Here's how the part is built. I have some questions about the finished solid (model axes, mm). Face numbers are marked on the shaded views. A direction names the side the tool comes from. Round coordinates to 2 decimals unless told otherwise and drop trailing zeros. Write each loop counter-clockwise with the first axis right and the second up, starting at its lowest first coordinate (ties: lowest second). Pieces come first, ordered by that corner, then holes. Notation, with made-up numbers: (38, 25) - (94, 25) arc R31 ccw to (94, 54) - close; hole circle Ø5 at (-11, -24.75). An arc over 180 degrees is marked (long way). Use one line per item in the form item = value. Start each with the question number.
1. Will this pin go through, and if not, where does the flat tip stop? pin 1 (10 mm diameter, centred on x = 6.5, z = 16, fed in from +Y).
2. Which directions (+Z, -Z, +X, -X, +Y, -Y) give clear straight access to the entire face, cutting with the end or side of a thin tool? Please do the marked faces 4 and 5.
3. I want a section at B-B, the plane z = 6. List the corners of the cut face in (x, y) for me.
4. I want a section at C-C, the plane x = -8.5. List the corners of the cut face in (y, z) for me, plus the area to 3 significant figures.
5. If I drill on line 1 along Z through (x, y) = (-1, 27), over which ranges is the centre line in solid material (lowest first)?
6. I want a section at D-D, the plane y = -30.5. List the corners of the cut face in (x, z) for me, plus the area to 3 significant figures.
7. I want a section at A-A, the plane y = 59.5. List the corners of the cut face in (x, z) for me, plus the area to 3 significant figures.
8. We'd pull the mould along Z, two halves only. Please class the marked faces 1, 2 and 3: +Z half, -Z half, draft (parallel to the pull), parting line (faces both ways), or undercut.
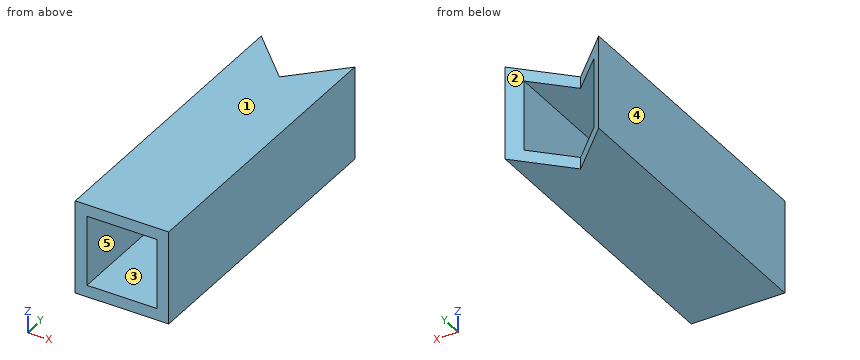
```python
from build123d import *

# Parameters (mm, degrees)
SKETCH1_W               = 50.8
SKETCH1_H               = 50.8
SKETCH1_W_2             = 38.1
SKETCH1_H_2             = 38.1
BOSS_EXTRUDE1_DEPTH     = 82.55
CUT_EXTRUDE1_DEPTH      = 1
CUT_EXTRUDE1_DEPTH_BACK = 51.8


with BuildPart() as part:
    # Sketch1 → Boss-Extrude1 (new body, symmetric)
    with BuildSketch(Plane(origin=(0, 0, 0), x_dir=(1, 0, 0), z_dir=(0, 1, 0))):
        Rectangle(SKETCH1_W, SKETCH1_H)
        Rectangle(SKETCH1_W_2, SKETCH1_H_2, mode=Mode.SUBTRACT)
    extrude(amount=BOSS_EXTRUDE1_DEPTH, both=True)

    # Sketch3 → Cut-Extrude1 (cut, two sides)
    with BuildSketch(Plane.XY.offset(25.4)) as cut_extrude1_sk:
        Polygon((-276.760445395, 333.910445395), (-25.4, 82.55), (0, 57.15), (25.4, 82.55), (276.760445395, 333.910445395), (276.760445395, 1044.865147239), (-276.760445395, 1044.865147239), align=None)
    extrude(amount=CUT_EXTRUDE1_DEPTH, mode=Mode.SUBTRACT)
    extrude(cut_extrude1_sk.sketch, amount=-CUT_EXTRUDE1_DEPTH_BACK, mode=Mode.SUBTRACT)


solid = part.part
```
Model answer:
q1.pin_1 = 67.61
q2.face_4 = +Z, -Z, -X, +Y, -Y
q2.face_5 = +Y, -Y
q3.outline = (-25.4, -82.55) - (-19.05, -82.55) - (-19.05, 76.2) - (-25.4, 82.55) - close; (19.05, -82.55) - (25.4, -82.55) - (25.4, 82.55) - (19.05, 76.2) - close
q4.outline = (-82.55, -25.4) - (65.65, -25.4) - (65.65, -19.05) - (-82.55, -19.05) - close; (-82.55, 19.05) - (65.65, 19.05) - (65.65, 25.4) - (-82.55, 25.4) - close
q4.area = 1,880 mm2
q5.line_1 = -25.4 to -19.05, 19.05 to 25.4
q6.outline = (-25.4, -25.4) - (25.4, -25.4) - (25.4, 25.4) - (-25.4, 25.4) - close; hole (-19.05, -19.05) - (19.05, -19.05) - (19.05, 19.05) - (-19.05, 19.05) - close
q6.area = 1,130 mm2
q7.outline = (-25.4, -25.4) - (-2.35, -25.4) - (-2.35, -19.05) - (-19.05, -19.05) - (-19.05, 19.05) - (-2.35, 19.05) - (-2.35, 25.4) - (-25.4, 25.4) - close; (2.35, -25.4) - (25.4, -25.4) - (25.4, 25.4) - (2.35, 25.4) - (2.35, 19.05) - (19.05, 19.05) - (19.05, -19.05) - (2.35, -19.05) - close
q7.area = 1,070 mm2
q8.face_1 = +Z half
q8.face_2 = draft
q8.face_3 = undercut
